from build123d import *

# Parameters (mm, degrees)
SKETCH_R          = 1.5
PAD_DEPTH         = 2
SKETCH001_W       = 2
SKETCH001_H       = 15
PAD001_DEPTH      = 7
PAD001_DEPTH_BACK = 2
FILLET_R          = 1
FILLET001_R       = 0.9


with BuildPart() as part:
    # Sketch → Pad (new body)
    with BuildSketch(Plane.XY):
        with BuildLine():
            ThreePointArc((-7.5, 3), (-10.5, 0), (-7.5, -3))
            Line((-7.5, -3), (7.5, -3))
            ThreePointArc((7.5, -3), (10.5, 0), (7.5, 3))
            Line((-7.5, 3), (7.5, 3))
        make_face()
        with Locations((-7.5, 0)):
            Circle(SKETCH_R, mode=Mode.SUBTRACT)
        with Locations((7.5, 0)):
            Circle(SKETCH_R, mode=Mode.SUBTRACT)
    extrude(amount=PAD_DEPTH)

    # Sketch001 (on Face8 of Pad) → Pad001 (join, two sides)
    with BuildSketch(Plane.XY.offset(2)) as pad001_sk:
        with Locations((0, 4.5)):
            Rectangle(SKETCH001_W, SKETCH001_H)
    extrude(amount=PAD001_DEPTH)
    extrude(pad001_sk.sketch, amount=-PAD001_DEPTH_BACK)

    # Fillet
    fillet_edges = [part.edges().sort_by_distance(p)[0] for p in [
        (1, 0, 2),
        (-1, 0, 2),
        (0, -3, 9),
        (0, 12, 9),
        (0, 12, 0),
        (1, 3, 1),
        (-1, 3, 1),
    ]]
    fillet(fillet_edges, radius=FILLET_R)

    # Fillet001
    fillet001_edges = [part.edges().sort_by_distance(p)[0] for p in [
        (1, 11.707107, 8.707107),
    ]]
    fillet(fillet001_edges, radius=FILLET001_R)


solid = part.part
Can you work these out from the model? Positions are in its coordinate system, mm. A direction names the side the tool comes from. Give positions to 0.01 mm unless a question says otherwise; leave off trailing zeros. Loops run counter-clockwise (first coordinate to the right, second up) from the corner with the lowest first, then second, coordinate; pieces in that order, holes last. Notation, with made-up numbers: (23, 15.5) - (62, 15.5) arc R22 cw to (62, 47.5) - close; hole circle Ø3 at (-26, -8.75). An arc over 180 degrees is marked (long way). Return JSON: item names as keys, results as strings.
1. I'm going to push flat-ended pins straight in: pin 1 Ø4.5 at (x, y) = (-7.5, -1) entering from +Z; pin 2 Ø1 at (x, y) = (-1, 4) entering from +Z; pin 3 Ø3.5 at (y, z) = (6.5, 4.5) entering from +X; pin 4 Ø3 at (x, y) = (-4.5, 5) entering from +Z. Where does each tip first touch, or does it pass through?
Output values:
{"pin 1": "stops at z = 2", "pin 2": "stops at z = 8.91", "pin 3": "stops at x = 1", "pin 4": "passes through"}
2. For faces 4 (the face through (0, -3, 2)), 5 (the face through (4.79, 2.74, 0.27)), 6 (the face through (4.71, -2.73, 1.74)), 7 (the face through (-1, 4, 5)), which set-ups out of +Z, -Z, +X, -X, +Y, -Y let a thin tool reach every point of the face, with its end or its side?
Output values:
{"face 4": "+Z, -Z, +X, -X, -Y", "face 5": "-Z, +X, +Y", "face 6": "+Z, +X, -Y", "face 7": "+Z, -X, +Y"}
3. If I drill on line 1 (X direction, y = 0.5, z = 1.75); line 2 (Y direction, x = -7.5, z = 1.05); line 3 (X direction, y = 3.75, z = 5.25), over which ranges is the centre line in solid material (lowest first)?
Output values:
{"line 1": "x = -10.18 to -8.91, -6.09 to 6.09, 8.91 to 10.18", "line 2": "y = -3 to -1.5, 1.5 to 3", "line 3": "x = -1 to 1"}
4. We'd pull the mould along Y, two halves only. Please class faces 1 (the face through (-4.71, 2.73, 1.74)), 2 (the face through (1, 4, 5)), 3 (the face through (6, 0, 1)): +Y half, -Y half, draft (parallel to the pull), parting line (faces both ways), or undercut.
Output values:
{"face 1": "+Y half", "face 2": "draft", "face 3": "undercut"}
5. I want a section at B-B on x = 4.25. Please give me the cut outline in (y, z).
Output values:
{"outline": "(-3, 0.9) arc R0.9 ccw to (-2.1, 0) - (2.1, 0) arc R0.9 ccw to (3, 0.9) - (3, 1.1) arc R0.9 ccw to (2.1, 2) - (-2.1, 2) arc R0.9 ccw to (-3, 1.1) - close"}
6. I want a section at A-A on y = 0. Please give me the cut outline in (x, z).
Output values:
{"outline": "(-10.5, 0.9) arc R0.9 ccw to (-9.6, 0) - (-9, 0) - (-9, 2) - (-9.6, 2) arc R0.9 ccw to (-10.5, 1.1) - close; (-6, 0) - (6, 0) - (6, 2) - (2, 2) arc R1 cw to (1, 3) - (1, 8.1) arc R0.9 ccw to (0.1, 9) - (-0.1, 9) arc R0.9 ccw to (-1, 8.1) - (-1, 3) arc R1 cw to (-2, 2) - (-6, 2) - close; (9, 0) - (9.6, 0) arc R0.9 ccw to (10.5, 0.9) - (10.5, 1.1) arc R0.9 ccw to (9.6, 2) - (9, 2) - close"}
7. I want a section at D-D on z = 0.5. Give the number of separate pieces and of enclosed holes in the cut face, and give its area (3 significant figures).
Output values:
{"separate pieces": "1", "enclosed holes": "2", "area": "116 mm²"}
8. I want a section at C-C on z = 4. Please give me the cut outline in (x, y), and give its area (3 significant figures).
Output values:
{"outline": "(-1, -2.1) arc R0.9 ccw to (-0.1, -3) - (0.1, -3) arc R0.9 ccw to (1, -2.1) - (1, 11.1) arc R0.9 ccw to (0.1, 12) - (-0.1, 12) arc R0.9 ccw to (-1, 11.1) - close", "area": "29.3 mm²"}
